Geometry: see drawing. Coordinates: mm, zero at the bounding-box minimum. Round coordinates to 2 decimals unless told otherwise and drop trailing zeros. Write each loop counter-clockwise with the first axis right and the second up, starting at its lowest first coordinate (ties: lowest second). Pieces come first, ordered by that corner, then holes. Notation, with made-up numbers: (-5.75, 44.25) -> (21.25, 44.25) arc R34 ccw to (21.25, 76.25) -> close; hole circle Ø1 at (-0.5, 82.5). An arc over 180 degrees is marked (long way). Write item = value, one per line. Start each with the question number.
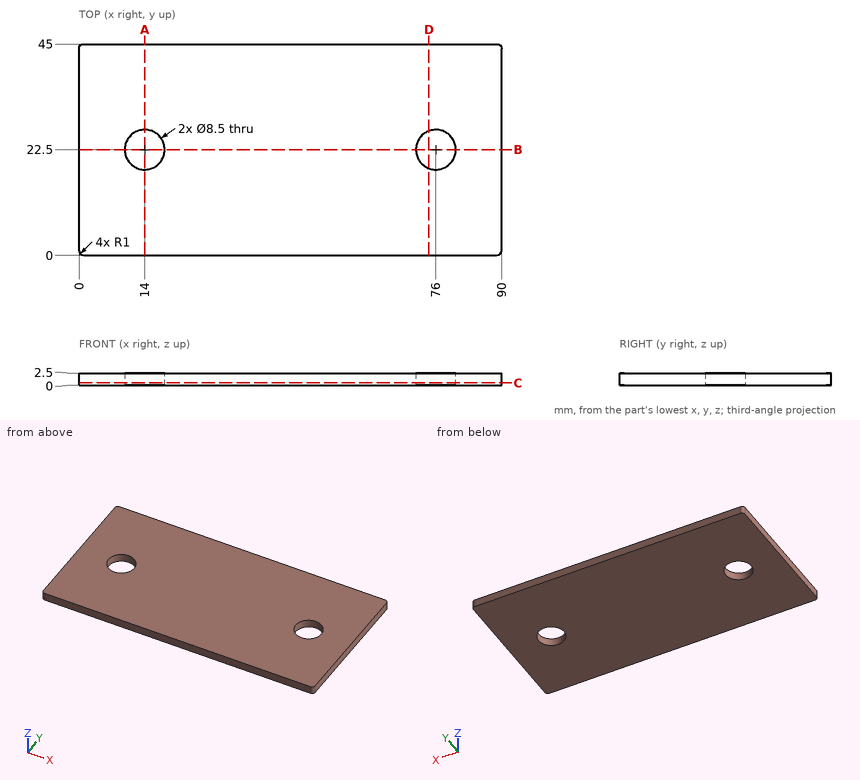
1. Section B-B (y = 22.5). Output: boundary loops of the cut face in (x, z).
2. Section D-D (x = 74.5). Output: boundary loops of the cut face in (y, z), then the cut area to 3 significant figures.
3. Section C-C (z = 0.45). Output: boundary loops of the cut face in (x, y).
4. Section A-A (x = 14). Output: boundary loops of the cut face in (y, z), then the cut area to 4 significant figures.
5. Line query: line 1 along Y through (x, z) = (76, 1.4); line 2 along X through (y, z) = (19, 0.6); line 3 along X through (y, z) = (19.5, 1.25). Output: solid intervals per line, ascending.
Check sheet entries:
q1.outline = (0, 0) -> (9.75, 0) -> (9.75, 2.5) -> (0, 2.5) -> close; (18.25, 0) -> (71.75, 0) -> (71.75, 2.5) -> (18.25, 2.5) -> close; (80.25, 0) -> (90, 0) -> (90, 2.5) -> (80.25, 2.5) -> close
q2.outline = (0, 0) -> (18.52, 0) -> (18.52, 2.5) -> (0, 2.5) -> close; (26.48, 0) -> (45, 0) -> (45, 2.5) -> (26.48, 2.5) -> close
q2.area = 92.6 mm2
q3.outline = (0, 1) arc R1 ccw to (1, 0) -> (89, 0) arc R1 ccw to (90, 1) -> (90, 44) arc R1 ccw to (89, 45) -> (1, 45) arc R1 ccw to (0, 44) -> close; hole circle Ø8.5 at (14, 22.5); hole circle Ø8.5 at (76, 22.5)
q4.outline = (0, 0) -> (18.25, 0) -> (18.25, 2.5) -> (0, 2.5) -> close; (26.75, 0) -> (45, 0) -> (45, 2.5) -> (26.75, 2.5) -> close
q4.area = 91.25 mm2
q5.line_1 = 0 to 18.25, 26.75 to 45
q5.line_2 = 0 to 11.59, 16.41 to 73.59, 78.41 to 90
q5.line_3 = 0 to 10.99, 17.01 to 72.99, 79.01 to 90
